Model file for the job. Use its own axes, mm. A direction names the side the tool comes from. Round coordinates to 2 decimals unless told otherwise and drop trailing zeros. Order: outer loops, then holes, each group sorted by start corner. A loop starts at its lowest first (then second) coordinate and runs counter-clockwise, first axis right, second up. Notation, with made-up numbers: M -33,42.5 L -4,42.5 A18 cw -4,65.5 Z; hole C 60.5,42.5 d2. An arc over 180 degrees is marked long. Return JSON: item names as keys, results as strings. Group by question number.
Item 1: Pin check, flat tips, straight feed: pin 1 Ø2.5 at (x, y) = (-21.75, 21.75) entering from +Z; pin 2 Ø4.5 at (x, y) = (0.5, -25) entering from +Z; pin 3 Ø2 at (y, z) = (2, 40) entering from -X. Stop position of each tip, or through.
Item 2: Slice it at A-A on x = 0. Write the cut outline in (y, z).
Item 3: Slice it at C-C on z = 46. Write the cut outline in (x, y), then the cut area to 3 significant figures.
Item 4: Slice it at B-B on y = 0. Write the cut outline in (x, z).
Item 5: Probe line 1 along Y through (x, z) = (-21.75, 6); line 2 along Z through (x, y) = (-21, 17.5); line 3 along Y through (x, z) = (0, 8.25). List the from-to ranges inside material, lowest first.
Item 6: Slice it at D-D on z = 28.5. Write the cut outline in (x, y).
Item 7: Pull direction Z, two halves, no side cores. Call faces 1 (the face through (22, -22, 10)), 2 (the face through (-5, -26, 3)), 3 (the face through (-26.32, 26.25, 10.14)): pulls with the +Z half, pulls with the -Z half, needs draft (parallel to the pull), parting line crosses it, or undercut.
Item 8: Which spindle directions (+Z, -Z, +X, -X, +Y, -Y) get a long thin tool onto all of the face, cutting with end or side? Do faces 4 (the face through (0, -26, 5)), 5 (the face through (-5.85, -26.36, 29.01)), 6 (the face through (-20.64, -20.74, 4.93)), 7 (the face through (-27.75, 0, 10)). Say none if no direction does.
from build123d import *

# Parameters (mm, degrees)
SKETCH_1_W          = 55.5
SKETCH_1_H          = 55.5
EXTRUDE_1_DEPTH     = 20
SKETCH_2_R          = 27
EXTRUDE_3_DEPTH     = 20
SKETCH_3_R          = 26
EXTRUDE_6_DEPTH     = 15
FILLET_1_R          = 5
FILLET_2_R          = 2
FILLET_3_R          = 5
SKETCH_5_R          = 1.5
CUT_EXTRUDE_1_DEPTH = 10
SKETCH_6_W          = 5
SKETCH_6_H          = 4
CUT_EXTRUDE_2_DEPTH = 4


with BuildPart() as part:
    # 草图1 → 凸台-拉伸1 (new body)
    with BuildSketch(Plane.XY):
        Rectangle(SKETCH_1_W, SKETCH_1_H)
    extrude(amount=EXTRUDE_1_DEPTH)

    # 草图2 → 凸台-拉伸3 (add)
    with BuildSketch(Plane.XY.offset(20)):
        Circle(SKETCH_2_R)
    extrude(amount=EXTRUDE_3_DEPTH)

    # 草图3 → 凸台-拉伸6 (add)
    with BuildSketch(Plane.XY.offset(40)):
        Circle(SKETCH_3_R)
    extrude(amount=EXTRUDE_6_DEPTH)

    # 圆角1
    fillet_1_edges = [part.edges().sort_by_distance(p)[0] for p in [
        (-26, 0, 55),
    ]]
    fillet(fillet_1_edges, radius=FILLET_1_R)

    # 圆角2
    # the kernel refuses this fillet: 2 mm, written as the material it takes off along each edge
    with BuildSketch(Plane(origin=(0, 0, 40), x_dir=(1, 0, 0), z_dir=(0, -1, 0))) as fillet_2_piece_1:
        with BuildLine():
            CenterArc((25, -1.732050808), FILLET_2_R, 0, 60)
            Line((27, -1.732050808), (27.04, -1.732050808))
            Line((27.04, -1.732050808), (27.04, 0))
            Line((27.04, 0), (27, 0.04))
            ThreePointArc((27, 0.04), (26.5, 0.04), (26.02, 0.034641016))
            Line((26.02, 0.034641016), (26, 0))
        make_face()
    revolve(axis=Axis((0, 0, 40), (0, 0, 1)), mode=Mode.SUBTRACT)

    # 圆角3
    fillet_3_edges = [part.edges().sort_by_distance(p)[0] for p in [
        (-27.75, 27.75, 10),
        (27.75, 27.75, 10),
        (27.75, -27.75, 10),
        (-27.75, -27.75, 10),
    ]]
    fillet(fillet_3_edges, radius=FILLET_3_R)

    # 草图5 → 切除-拉伸1 (cut)
    with BuildSketch(Plane(origin=(0, 0, 0), x_dir=(-1, 0, 0), z_dir=(0, 0, -1))):
        Circle(SKETCH_5_R)
        with Locations((-21.75, 21.75)):
            Circle(SKETCH_5_R)
        with Locations(Location((21.75, 21.75, 0), (0, 0, 180))):
            Circle(SKETCH_5_R)
        with Locations((21.75, -21.75)):
            Circle(SKETCH_5_R)
        with Locations(Location((-21.75, -21.75, 0), (0, 0, 180))):
            Circle(SKETCH_5_R)
    extrude(amount=-CUT_EXTRUDE_1_DEPTH, mode=Mode.SUBTRACT)

    # 草图6 → 切除-拉伸2 (cut)
    with BuildSketch(Plane.XZ.offset(27.75)):
        with Locations((-2.5, 3)):
            Rectangle(SKETCH_6_W, SKETCH_6_H)
        with Locations((2.5, 3)):
            Rectangle(SKETCH_6_W, SKETCH_6_H)
    extrude(amount=-CUT_EXTRUDE_2_DEPTH, mode=Mode.SUBTRACT)


solid = part.part
Output values:
{
 "1": {"pin 1": "z = 20", "pin 2": "z = 54.68", "pin 3": "x = -26.79"},
 "2": {"outline": "M -27.75,0 L -1.5,0 L -1.5,10 L 1.5,10 L 1.5,0 L 27.75,0 L 27.75,20 L 27,20 L 27,38.27 A2 ccw 26,40 L 26,50 A5 ccw 21,55 L -21,55 A5 ccw -26,50 L -26,40 A2 ccw -27,38.27 L -27,20 L -27.75,20 L -27.75,5 L -23.75,5 L -23.75,1 L -27.75,1 Z"},
 "3": {"outline": "C 0,0 d52", "area": "2,120 mm²"},
 "4": {"outline": "M -27.75,0 L -1.5,0 L -1.5,10 L 1.5,10 L 1.5,0 L 27.75,0 L 27.75,20 L 27,20 L 27,38.27 A2 ccw 26,40 L 26,50 A5 ccw 21,55 L -21,55 A5 ccw -26,50 L -26,40 A2 ccw -27,38.27 L -27,20 L -27.75,20 Z"},
 "5": {"line 1": "-27.75 to -23.25, -20.25 to 20.25, 23.25 to 27.75", "line 2": "0 to 20", "line 3": "-27.75 to -1.5, 1.5 to 27.75"},
 "6": {"outline": "C 0,0 d54"},
 "7": {"face 1": "pulls with the -Z half", "face 2": "undercut", "face 3": "needs draft"},
 "8": {"face 4": "-Y", "face 5": "+Z", "face 6": "-Z", "face 7": "+Z, -Z, -X, +Y, -Y"}
}
